For this review, use the dimensioned drawing (mm, ordinates from the lowest corner) and the shaded views. A direction names the side the tool comes from. Give positions to 0.01 mm unless a question says otherwise; leave off trailing zeros. Order: outer loops, then holes, each group sorted by start corner. A loop starts at its lowest first (then second) coordinate and runs counter-clockwise, first axis right, second up. Notation, with made-up numbers: (67, 39.5) - (86, 39.5) arc R36 cw to (86, 78.5) - close; hole circle Ø7 at (68.5, 22). An arc over 180 degrees is marked (long way). Use a Markdown table: item, result. Add a question column.
1) We need section A-A on y = 5.5. Write out the cut boundary in (x, z), then the cut area to 3 significant figures.
2) Clearance check with flat-ended pins moving along their axes: P1, Ø2.5, axis at x = 5.5, y = 36.5, coming from the +Z side; P2, Ø6, axis at x = 11.5, y = 16, coming from the +Z side; P3, Ø1.4, axis at y = 20.5, z = 51.5, coming from the +X side. State where each tip first meets the part, or that it passes through.
3) We need section D-D on x = 21. Write out the cut boundary in (y, z), then the cut area to 3 significant figures.
4) Mouldability with a two-part tool opening along Y and no side actions: class the marked faces 3, 4 and 5 as released by +Y, released by -Y, zero draft, split by the parting line, or undercut.
5) Machinability: for the marked faces 1 and 2, which of the approach directions +Z, -Z, +X, -X, +Y, -Y give a long, thin tool a straight path to every point of the face, cutting with its end or side? Answer none if there is none.
6) Wall thickness on L1, parallel to X at y = 5.5, z = 20; L2, parallel to X at y = 5, z = 23: over which ranges is each line inside the solid? List them lowest first.
7) We need section C-C on z = 37.5. Write out the cut boundary in (x, y), then the cut area to 3 significant figures.
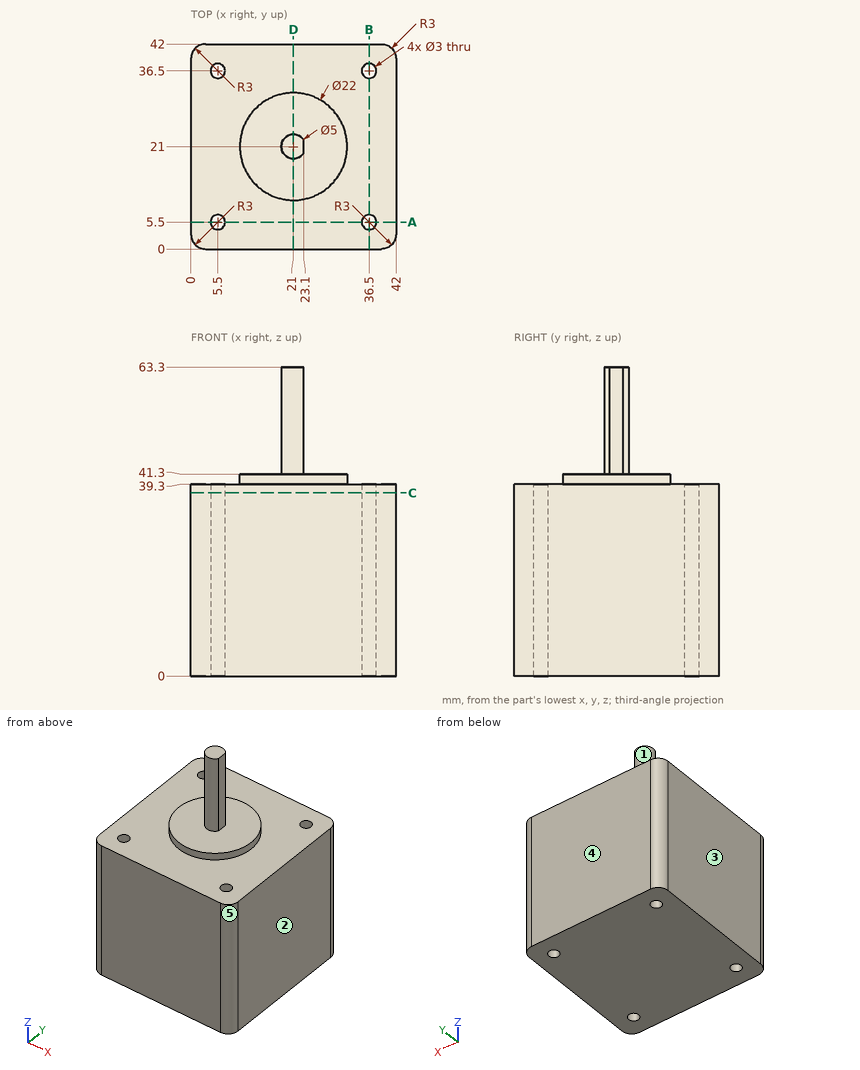
Checked values:
| question | item | result |
|---|---|---|
| 1 | outline | (0, 0) - (4, 0) - (4, 39.3) - (0, 39.3) - close; (7, 0) - (35, 0) - (35, 39.3) - (7, 39.3) - close; (38, 0) - (42, 0) - (42, 39.3) - (38, 39.3) - close |
| 1 | area | 1,410 mm² |
| 2 | P1 | through |
| 2 | P2 | z = 41.3 |
| 2 | P3 | x = 23.1 |
| 3 | outline | (0, 0) - (42, 0) - (42, 39.3) - (32, 39.3) - (32, 41.3) - (23.5, 41.3) - (23.5, 63.3) - (18.5, 63.3) - (18.5, 41.3) - (10, 41.3) - (10, 39.3) - (0, 39.3) - close |
| 3 | area | 1,800 mm² |
| 4 | face 3 | zero draft |
| 4 | face 4 | released by +Y |
| 4 | face 5 | released by -Y |
| 5 | face 1 | +Z |
| 5 | face 2 | +Z, -Z, +X, +Y, -Y |
| 6 | L1 | 0 to 4, 7 to 35, 38 to 42 |
| 6 | L2 | 0 to 4.09, 6.91 to 35.09, 37.91 to 42 |
| 7 | outline | (0, 3) arc R3 ccw to (3, 0) - (39, 0) arc R3 ccw to (42, 3) - (42, 39) arc R3 ccw to (39, 42) - (3, 42) arc R3 ccw to (0, 39) - close; hole circle Ø3 at (5.5, 5.5); hole circle Ø3 at (5.5, 36.5); hole circle Ø3 at (36.5, 5.5); hole circle Ø3 at (36.5, 36.5) |
| 7 | area | 1,730 mm² |
